Drawing for the job (mm, zero at the part's lowest x, y, z). A direction names the side the tool comes from. Round coordinates to 2 decimals unless told otherwise and drop trailing zeros. Write each loop counter-clockwise with the first axis right and the second up, starting at its lowest first coordinate (ties: lowest second). Pieces come first, ordered by that corner, then holes. Notation, with made-up numbers: M 63,81 L 90,81 A18 cw 90,108 Z; hole C 19.25,33.5 d6. An arc over 180 degrees is marked long. Use a Markdown table: item, result. Add a question column.
1) Wall check: probe 1 along Y at (x, z) = (85, 40); probe 2 along X at (y, z) = (54, 63.5); probe 3 along Z at (x, y) = (72.5, 48). Give the ranges that are in metal, low to high.
2) Two-plate mould, pull along Y, no slides. Class the marked faces 3, 4, 5 and 6: released by +Y, released by -Y, zero draft, split by the parting line, or undercut.
3) Slice it at C-C on z = 47.5. Write the cut outline in (x, y), plus the area to 3 significant figures.
4) Which spindle directions (+Z, -Z, +X, -X, +Y, -Y) get a long thin tool onto all of the face, cutting with end or side? Do the marked faces 1 and 2. Say none if no direction does.
5) Slice it at D-D on y = 61. Write the cut outline in (x, z).
6) Drop flat-ended pins along their axis: P1, Ø3, axis at x = 111, y = 19.5, coming from the +Z side; P2, Ø11, axis at x = 6, y = 41.5, coming from the +Z side. Give the stop position or say it passes through.
7) Slice it at A-A on y = 39.5. Write the cut outline in (x, z).
8) Slice it at B-B on x = 70.5. Write the cut outline in (y, z), plus the area to 3 significant figures.
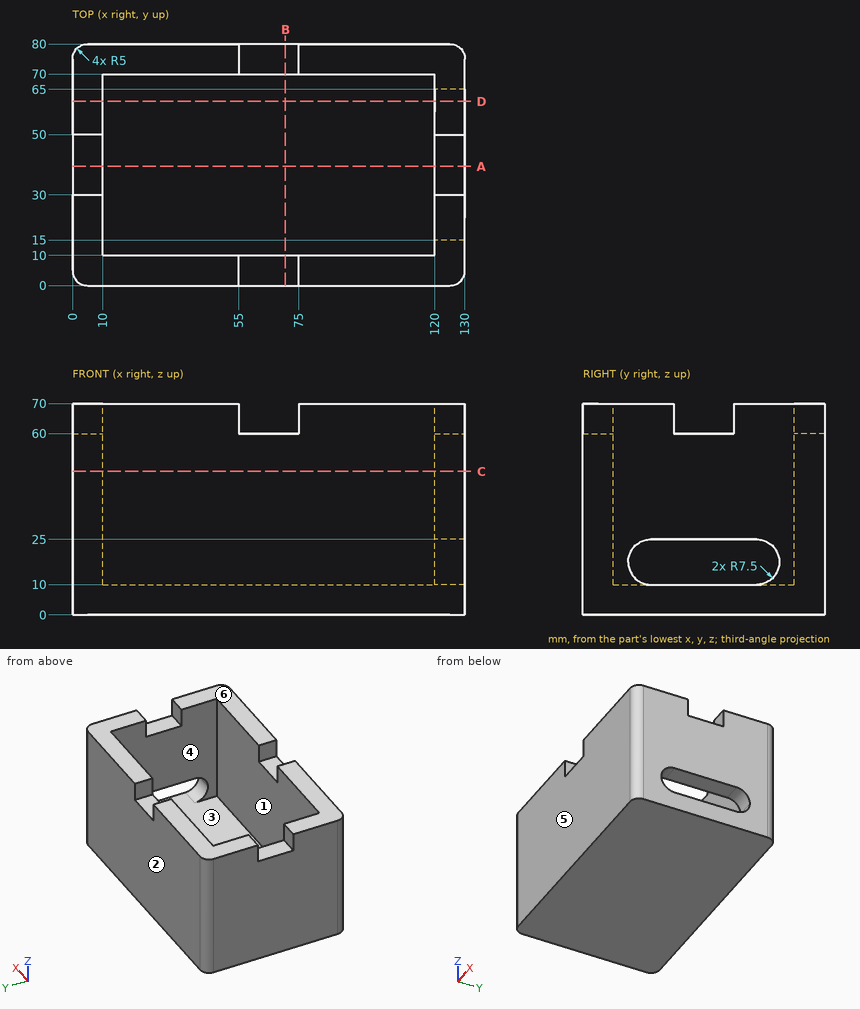
Entries:
| question | item | result |
|---|---|---|
| 1 | probe 1 | y = 0 to 10, 70 to 80 |
| 1 | probe 2 | x = 0 to 10, 120 to 130 |
| 1 | probe 3 | z = 0 to 10 |
| 2 | face 3 | undercut |
| 2 | face 4 | undercut |
| 2 | face 5 | released by -Y |
| 2 | face 6 | zero draft |
| 3 | outline | M 0,5 A5 ccw 5,0 L 125,0 A5 ccw 130,5 L 130,75 A5 ccw 125,80 L 5,80 A5 ccw 0,75 Z; hole M 10,10 L 120,10 L 120,70 L 10,70 Z |
| 3 | area | 3,780 mm^2 |
| 4 | face 1 | +Z |
| 4 | face 2 | +Z, -Z, +X, -X, +Y |
| 5 | outline | M 0,0 L 130,0 L 130,10.87 L 120,10.87 L 120,10 L 10,10 L 10,70 L 0,70 Z; M 120,24.13 L 130,24.13 L 130,70 L 120,70 Z |
| 6 | P1 | stops at z = 10 |
| 6 | P2 | stops at z = 60 |
| 7 | outline | M 0,0 L 130,0 L 130,10 L 10,10 L 10,60 L 0,60 Z; M 120,25 L 130,25 L 130,60 L 120,60 Z |
| 8 | outline | M 0,0 L 80,0 L 80,60 L 70,60 L 70,10 L 10,10 L 10,60 L 0,60 Z |
| 8 | area | 1,800 mm^2 |
